Geometry check sheet. Reference: the model listing, model coordinates, mm. Face numbers are marked on the shaded views. A direction names the side the tool comes from. Round coordinates to 2 decimals unless told otherwise and drop trailing zeros. Write each loop counter-clockwise with the first axis right and the second up, starting at its lowest first coordinate (ties: lowest second). Pieces come first, ordered by that corner, then holes. Notation, with made-up numbers: M 27,48.25 L 64,48.25 A24 cw 64,66.25 Z; hole C 3,-26 d3. An arc over 180 degrees is marked long. Put each result on its own line as item: value. Start each with the question number.
(1) Section check C-C on y = 81. Record the cut outline in (x, z), then the cut area to 3 significant figures.
(2) Section check A-A on z = -9.75. Record the cut outline in (x, y), then the cut area to 3 significant figures.
(3) Material ranges on probe 1 along Z at (x, y) = (3.25, 88); probe 2 along Z at (x, y) = (12.25, 110.5), recorded low to high.
(4) Section check B-B on x = 2. Record the cut outline in (y, z), then the cut area to 3 significant figures.
(5) Tool access check on the marked faces 1 and 2. Record the directions out of +Z, -Z, +X, -X, +Y, -Y that give a thin tool (end or side, any length) a straight path to the whole face; none if there is none.
(6) Mould release check, pull along X, two halves, no side actions. Record for the marked faces 3, 4 and 5: pulls with the +X half, pulls with the -X half, needs draft (parallel to the pull), parting line crosses it, or undercut.
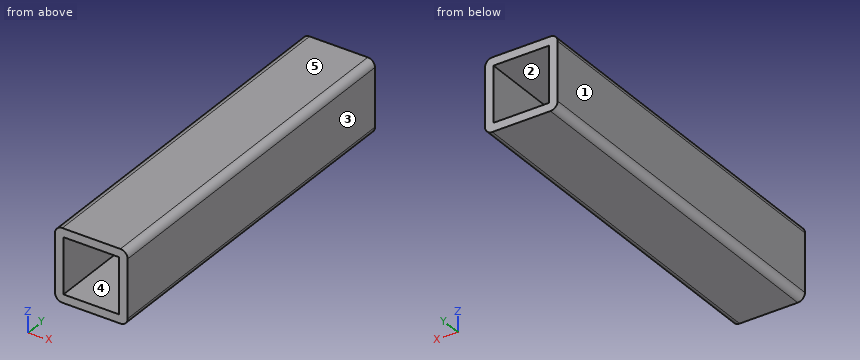
from build123d import *

# Parameters (mm, degrees)
SKETCH1_W           = 23
SKETCH1_H           = 23
BOSS_EXTRUDE1_DEPTH = 150


with BuildPart() as part:
    # Sketch1 → Boss-Extrude1 (new body)
    with BuildSketch(Plane(origin=(0, 0, 0), x_dir=(1, 0, 0), z_dir=(0, 1, 0))):
        with BuildLine():
            Line((12, 15), (-12, 15))
            ThreePointArc((-12, 15), (-14.121320344, 14.121320344), (-15, 12))
            Line((-15, 12), (-15, -12))
            ThreePointArc((-15, -12), (-14.121320344, -14.121320344), (-12, -15))
            Line((-12, -15), (12, -15))
            ThreePointArc((12, -15), (14.121320344, -14.121320344), (15, -12))
            Line((15, -12), (15, 12))
            ThreePointArc((15, 12), (14.121320344, 14.121320344), (12, 15))
        make_face()
        Rectangle(SKETCH1_W, SKETCH1_H, mode=Mode.SUBTRACT)
    extrude(amount=BOSS_EXTRUDE1_DEPTH)


solid = part.part
Answers follow:
1. outline: M -15,-12 A3 ccw -12,-15 L 12,-15 A3 ccw 15,-12 L 15,12 A3 ccw 12,15 L -12,15 A3 ccw -15,12 Z; hole M -11.5,-11.5 L 11.5,-11.5 L 11.5,11.5 L -11.5,11.5 Z
1. area: 363 mm^2
2. outline: M -15,0 L -11.5,0 L -11.5,150 L -15,150 Z; M 11.5,0 L 15,0 L 15,150 L 11.5,150 Z
2. area: 1,050 mm^2
3. probe 1: z = -15 to -11.5, 11.5 to 15
3. probe 2: z = -14.99 to 14.99
4. outline: M 0,-15 L 150,-15 L 150,-11.5 L 0,-11.5 Z; M 0,11.5 L 150,11.5 L 150,15 L 0,15 Z
4. area: 1,050 mm^2
5. face 1: +Z, -Z, -X, +Y, -Y
5. face 2: +Y, -Y
6. face 3: pulls with the +X half
6. face 4: undercut
6. face 5: needs draft
